from build123d import *

# Parameters (mm, degrees)
BOSS_EXTRUDE1_DEPTH = 3.175
SKETCH7_R           = 6.35
SKETCH7_R_2         = 1.778
CUT_EXTRUDE3_DEPTH  = 3.175
CUT_EXTRUDE4_REACH  = 98.387
SKETCH8_R           = 6.35
SKETCH8_R_2         = 1.778


with BuildPart() as part:
    # Sketch1 → Boss-Extrude1 (new body)
    with BuildSketch(Plane(origin=(0, 0, 0), x_dir=(1, 0, 0), z_dir=(0, 1, 0))):
        Polygon((0, 0), (-51.308, 0), (-51.308, -20.32), (-25.4, -20.32), (-25.4, -81.534), (0, -81.534), align=None)
    extrude(amount=BOSS_EXTRUDE1_DEPTH)

    # Sketch7 → Cut-Extrude3 (cut)
    with BuildSketch(Plane(origin=(0, 3.175, 0), x_dir=(1, 0, 0), z_dir=(0, 1, 0))):
        with Locations(Location((-12.7, -67.31, 0), (0, 0, 270))):
            Circle(SKETCH7_R)
        with Locations(Location((-5.785202787, -60.395202787, 0), (0, 0, 270))):
            Circle(SKETCH7_R_2)
        with Locations(Location((-5.785202787, -74.224797213, 0), (0, 0, 270))):
            Circle(SKETCH7_R_2)
        with Locations(Location((-19.614797213, -74.224797213, 0), (0, 0, 270))):
            Circle(SKETCH7_R_2)
        with Locations(Location((-19.614797213, -60.395202787, 0), (0, 0, 270))):
            Circle(SKETCH7_R_2)
    extrude(amount=-CUT_EXTRUDE3_DEPTH, mode=Mode.SUBTRACT)

    # Sketch8 → Cut-Extrude4 (cut, up to next)
    with BuildSketch(Plane(origin=(0, 3.175, 0), x_dir=(1, 0, 0), z_dir=(0, 1, 0)), mode=Mode.PRIVATE) as cut_extrude4_sk1:
        with Locations(Location((-41.148, -10.16, 0), (0, 0, 270))):
            Circle(SKETCH8_R)
    cut_extrude4_tool1 = extrude(cut_extrude4_sk1.sketch, amount=-CUT_EXTRUDE4_REACH, mode=Mode.PRIVATE) & part.part
    # Sketch8 → Cut-Extrude4 (cut, up to next)
    with BuildSketch(Plane(origin=(0, 3.175, 0), x_dir=(1, 0, 0), z_dir=(0, 1, 0)), mode=Mode.PRIVATE) as cut_extrude4_sk2:
        with Locations(Location((-48.062797213, -3.245202787, 0), (0, 0, 270))):
            Circle(SKETCH8_R_2)
    cut_extrude4_tool2 = extrude(cut_extrude4_sk2.sketch, amount=-CUT_EXTRUDE4_REACH, mode=Mode.PRIVATE) & part.part
    # Sketch8 → Cut-Extrude4 (cut, up to next)
    with BuildSketch(Plane(origin=(0, 3.175, 0), x_dir=(1, 0, 0), z_dir=(0, 1, 0)), mode=Mode.PRIVATE) as cut_extrude4_sk3:
        with Locations(Location((-34.233202787, -3.245202787, 0), (0, 0, 270))):
            Circle(SKETCH8_R_2)
    cut_extrude4_tool3 = extrude(cut_extrude4_sk3.sketch, amount=-CUT_EXTRUDE4_REACH, mode=Mode.PRIVATE) & part.part
    # Sketch8 → Cut-Extrude4 (cut, up to next)
    with BuildSketch(Plane(origin=(0, 3.175, 0), x_dir=(1, 0, 0), z_dir=(0, 1, 0)), mode=Mode.PRIVATE) as cut_extrude4_sk4:
        with Locations(Location((-34.233202787, -17.074797213, 0), (0, 0, 270))):
            Circle(SKETCH8_R_2)
    cut_extrude4_tool4 = extrude(cut_extrude4_sk4.sketch, amount=-CUT_EXTRUDE4_REACH, mode=Mode.PRIVATE) & part.part
    # Sketch8 → Cut-Extrude4 (cut, up to next)
    with BuildSketch(Plane(origin=(0, 3.175, 0), x_dir=(1, 0, 0), z_dir=(0, 1, 0)), mode=Mode.PRIVATE) as cut_extrude4_sk5:
        with Locations(Location((-48.062797213, -17.074797213, 0), (0, 0, 270))):
            Circle(SKETCH8_R_2)
    cut_extrude4_tool5 = extrude(cut_extrude4_sk5.sketch, amount=-CUT_EXTRUDE4_REACH, mode=Mode.PRIVATE) & part.part
    add(cut_extrude4_tool1.solids().sort_by_distance((-41.148, 3.175, 10.16))[0], mode=Mode.SUBTRACT)
    add(cut_extrude4_tool2.solids().sort_by_distance((-48.062797, 3.175, 3.245203))[0], mode=Mode.SUBTRACT)
    add(cut_extrude4_tool3.solids().sort_by_distance((-34.233203, 3.175, 3.245203))[0], mode=Mode.SUBTRACT)
    add(cut_extrude4_tool4.solids().sort_by_distance((-34.233203, 3.175, 17.074797))[0], mode=Mode.SUBTRACT)
    add(cut_extrude4_tool5.solids().sort_by_distance((-48.062797, 3.175, 17.074797))[0], mode=Mode.SUBTRACT)


solid = part.part
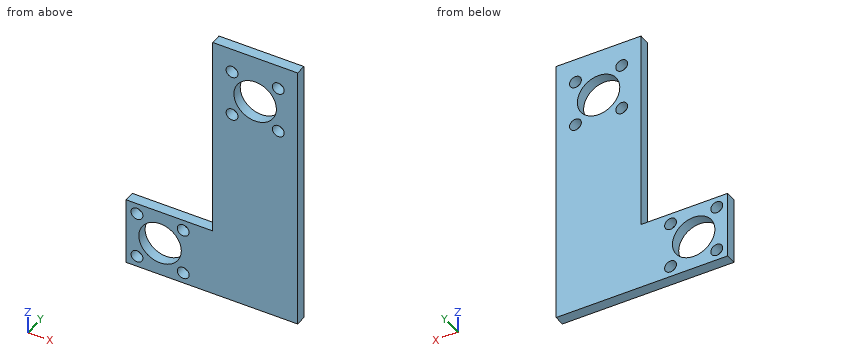
The listing builds one solid part. Answer for the finished solid, in the listing's coordinates (mm). Give positions to 0.01 mm unless a question says otherwise; leave off trailing zeros. Loops run counter-clockwise (first coordinate to the right, second up) from the corner with the lowest first, then second, coordinate; pieces in that order, holes last.
Item 1: A cutting plane is placed at C-C (y = 1.3). Give the number of separate pieces and of enclosed holes in the cut face, then the cut area to 3 significant figures.
Derived:
separate pieces: 1
enclosed holes: 10
area: 2,260 mm2
Item 2: A cutting plane is placed at B-B (x = -12.7). Give the vertices of the cut face in (y, z) (3 decimals).
Derived:
outline: (0, 0) - (3.175, 0) - (3.175, 60.96) - (0, 60.96) - close; (0, 73.66) - (3.175, 73.66) - (3.175, 81.534) - (0, 81.534) - close
Item 3: Find the intervals of material crossed by line 1 along Z through (x, y) = (-6, 1.05); line 2 along Z through (x, y) = (-18.5, 2.35); line 3 along Z through (x, y) = (-12.5, 2.5), in increasing order.
Derived:
line 1: z = 0 to 58.63, 62.16 to 72.46, 75.99 to 81.53
line 2: z = 0 to 59.01, 61.78 to 64.72, 69.9 to 72.84, 75.61 to 81.53
line 3: z = 0 to 60.96, 73.66 to 81.53
Item 4: Each of these flat-tipped pins is pushed along its axis until it touches: pin 1 Ø1 at (x, y) = (-31, 2) entering from +Z; pin 2 Ø1 at (y, z) = (2, 39.5) entering from -X; pin 3 Ø3 at (x, z) = (-5.79, 60.4) entering from -Y. Where does it stop, or does it pass through?
Derived:
pin 1: stops at z = 20.32
pin 2: stops at x = -25.4
pin 3: passes through
Item 5: A cutting plane is placed at D-D (z = 30). Give the vertices of the cut face in (x, y) (3 decimals).
Derived:
outline: (-25.4, 0) - (0, 0) - (0, 3.175) - (-25.4, 3.175) - close
Item 6: A cutting plane is placed at A-A (z = 67.31). Give the vertices of the cut face in (x, y) (3 decimals).
Derived:
outline: (-25.4, 0) - (-19.05, 0) - (-19.05, 3.175) - (-25.4, 3.175) - close; (-6.35, 0) - (0, 0) - (0, 3.175) - (-6.35, 3.175) - close
